Input: dimensioned drawing with shaded views. Units: mm. Origin: part minimum x, y, z. A direction names the side the tool comes from. Coordinates: 2 decimals unless noted, no trailing zeros. Order: outer loops, then holes, each group sorted by start corner. A loop starts at its lowest first (then second) coordinate and runs counter-clockwise, first axis right, second up. Notation, with made-up numbers: M -33.75,-2 L -13.75,-2 A30 cw -13.75,26 Z; hole C -10,0 d8. An arc over 180 degrees is marked long. Write item = value, one per line.
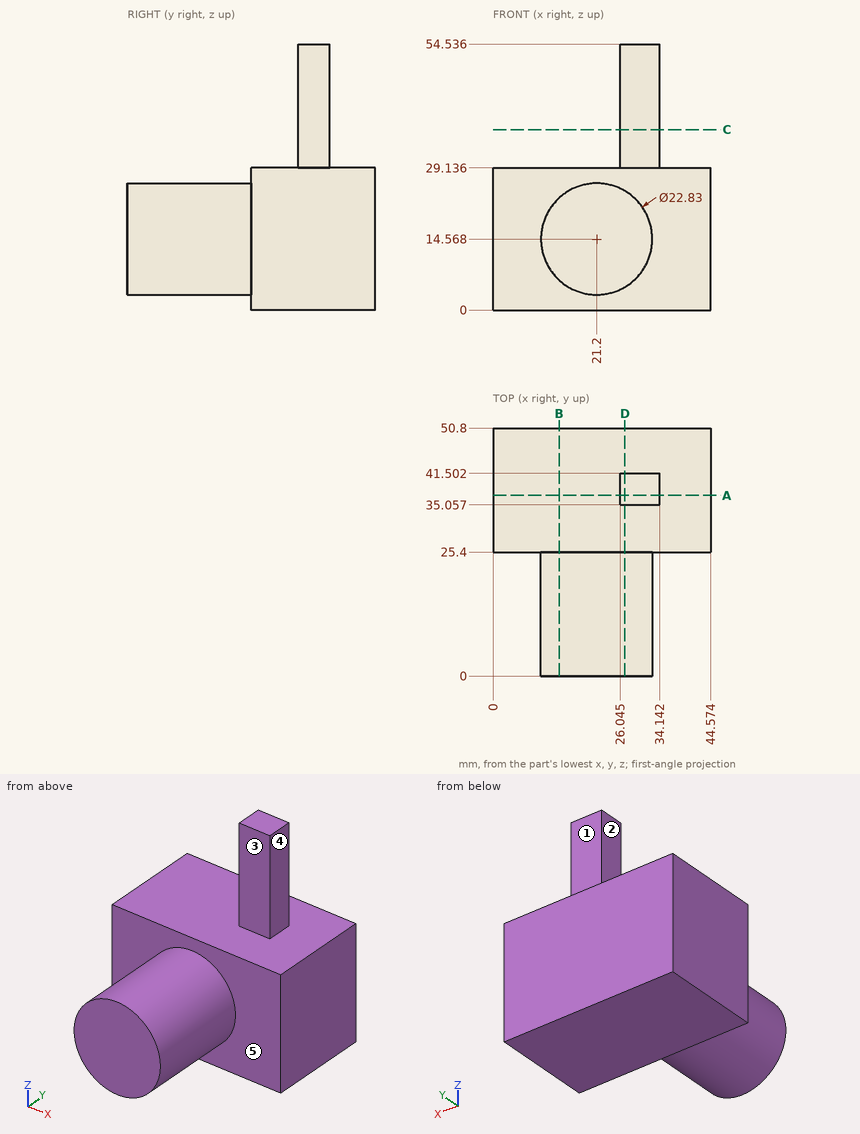
1) Section D-D, the plane x = 27. Return loops of the section in (y, z).
Numbers:
outline = M 0,4.74 L 25.4,4.74 L 25.4,0 L 50.8,0 L 50.8,29.14 L 41.5,29.14 L 41.5,54.54 L 35.06,54.54 L 35.06,29.14 L 25.4,29.14 L 25.4,24.4 L 0,24.4 Z
2) Section B-B, the plane x = 13.5. Return loops of the section in (y, z) (1 decimal), and give its area (3 significant figures).
Numbers:
outline = M 0,6.1 L 25.4,6.1 L 25.4,0 L 50.8,0 L 50.8,29.1 L 25.4,29.1 L 25.4,23 L 0,23 Z
area = 1,170 mm²
3) Line query: L1, parallel to Z at x = 12, y = 26; L2, parallel to X at y = 40.5, z = 31.5 (1 decimal); L3, parallel to Y at x = 31, z = 5.5. Output: solid intervals per line, ascending.
Numbers:
L1 = 0 to 29.14
L2 = 26 to 34.1
L3 = 25.4 to 50.8
4) Section C-C, the plane z = 37. Return loops of the section in (x, y) (1 decimal).
Numbers:
outline = M 26,35.1 L 34.1,35.1 L 34.1,41.5 L 26,41.5 Z
5) Set-up query: the marked faces 1, 2, 3, 4 and 5. Return all of +Z, -Z, +X, -X, +Y, -Y with unobstructed straight access to the full face (end or side cutting, diameter ignored); none if empty.
Numbers:
face_1 = +Z, +X, -X, +Y
face_2 = +Z, -X, +Y, -Y
face_3 = +Z, +X, -X, -Y
face_4 = +Z, +X, +Y, -Y
face_5 = -Y
6) Pin query (flat end, axial travel): pin 1 (3 mm diameter, centred on x = 22, y = 38, fed in from +Z); pin 2 (12 mm diameter, centred on x = 40, z = 23, fed in from -Y); pin 3 (1 mm diameter, centred on y = 16.5, z = 25.5, fed in from +X) (1 decimal); pin 4 (2 mm diameter, centred on x = 30.5, y = 33.5, fed in from -Z). Return the tip coordinate at first contact, or that it passes through.
Numbers:
pin_1 = 29.14
pin_2 = 25.4
pin_3 = 25.8
pin_4 = 0
7) Section A-A, the plane y = 37. Return loops of the section in (x, z) (1 decimal).
Numbers:
outline = M 0,0 L 44.6,0 L 44.6,29.1 L 34.1,29.1 L 34.1,54.5 L 26,54.5 L 26,29.1 L 0,29.1 Z
